```python
from build123d import *

# Parameters (mm, degrees)
SKETCH_1_R          = 15
EXTRUDE_1_DEPTH     = 5
SKETCH_3_R          = 22.5
EXTRUDE_3_DEPTH     = 4
SKETCH_6_R          = 10
CUT_EXTRUDE_2_DEPTH = 33.210246817
HOLE_WIZARD_M4_1_D  = 3.3


with BuildPart() as part:
    # 草图1 → 凸台-拉伸1 (new body)
    with BuildSketch(Plane(origin=(0, 0, 0), x_dir=(0, 0, -1), z_dir=(1, 0, 0))):
        Circle(SKETCH_1_R)
    extrude(amount=EXTRUDE_1_DEPTH)

    # 草图3 → 凸台-拉伸3 (add)
    with BuildSketch(Plane.ZY):
        Circle(SKETCH_3_R)
    extrude(amount=-EXTRUDE_3_DEPTH)

    # 草图6 → 切除-拉伸2 (cut, through all)
    with BuildSketch(Plane(origin=(5, 0, 0), x_dir=(0, 0, -1), z_dir=(1, 0, 0))):
        Circle(SKETCH_6_R)
    extrude(amount=-CUT_EXTRUDE_2_DEPTH, mode=Mode.SUBTRACT)

    # M4 螺纹孔1 (through all)
    with Locations(Plane(origin=(4, 0, 0), x_dir=(0, 0, -1), z_dir=(1, 0, 0))):
        with Locations((-13.258252147, 13.258252147), (13.258252147, 13.258252147), (13.258252147, -13.258252147), (-13.258252147, -13.258252147), (0, 0)):
            Hole(HOLE_WIZARD_M4_1_D / 2)


solid = part.part
```
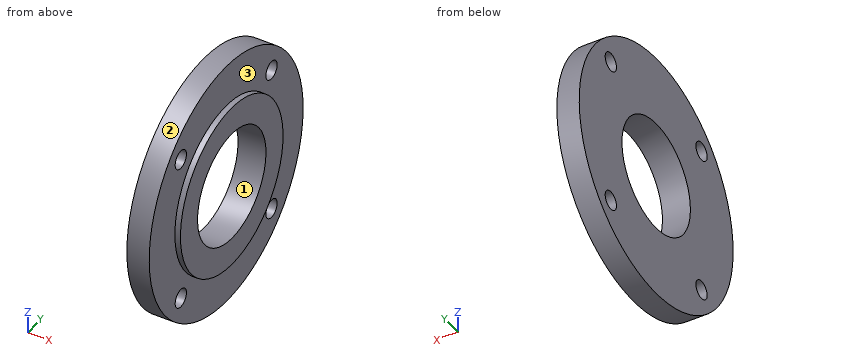
Input: part model. Units: mm. Frame: model coordinates. Face numbers are marked on the shaded views. Coordinates: 2 decimals unless noted, no trailing zeros. Loops run counter-clockwise (first coordinate to the right, second up) from the corner with the lowest first, then second, coordinate; pieces in that order, holes last. Notation, with made-up numbers: M -13,-39.75 L -7,-39.75 A26 cw -7,-24.75 Z; hole C 1,89.25 d7. An arc over 180 degrees is marked long. Answer in a Markdown table with one row per item.
1. Draft query along Y for the marked faces 1, 2 and 3. Return one class per face: pulls with the +Y half, pulls with the -Y half, needs draft (parallel to the pull), parting line crosses it, or undercut.
Response:
| item | result |
|---|---|
| face 1 | undercut |
| face 2 | parting line crosses it |
| face 3 | needs draft |
2. Section A-A, the plane y = 0. Output: boundary loops of the cut face in (x, z), then the cut area to 3 significant figures.
Response:
| item | result |
|---|---|
| outline | M 0,-22.5 L 4,-22.5 L 4,-15 L 5,-15 L 5,-10 L 0,-10 Z; M 0,10 L 5,10 L 5,15 L 4,15 L 4,22.5 L 0,22.5 Z |
| area | 110 mm2 |
3. Section D-D, the plane z = -11. Output: boundary loops of the cut face in (x, y).
Response:
| item | result |
|---|---|
| outline | M 0,-19.63 L 4,-19.63 L 4,-10.2 L 5,-10.2 L 5,10.2 L 4,10.2 L 4,19.63 L 0,19.63 Z |
4. First-contact query: pin 1 (5.5 mm diameter, centred on y = -13.26, z = 13.26, fed in from +X); pin 2 (1.5 mm diameter, centred on x = 2, y = -9, fed in from +Z). Flat tips, straight axial feed; report the tip coordinate or a pass-through.
Response:
| item | result |
|---|---|
| pin 1 | stops at x = 4 |
| pin 2 | stops at z = 20.93 |
5. Section C-C, the plane x = 1. Output: boundary loops of the cut face in (y, z).
Response:
| item | result |
|---|---|
| outline | C 0,0 d45; hole C -13.26,-13.26 d3.3; hole C -13.26,13.26 d3.3; hole C 0,0 d20; hole C 13.26,-13.26 d3.3; hole C 13.26,13.26 d3.3 |
6. Material intervals for line 1 (Y direction, x = 3.4, z = -14.5); line 2 (Y direction, x = 2, z = 0); line 3 (Y direction, x = 1.3, z = -8.5), sorted ascending.
Response:
| item | result |
|---|---|
| line 1 | y = -17.2 to -14.34, -12.17 to 12.17, 14.34 to 17.2 |
| line 2 | y = -22.5 to -10, 10 to 22.5 |
| line 3 | y = -20.83 to -5.27, 5.27 to 20.83 |
